Input: dimensioned drawing with shaded views. Units: mm. Origin: part minimum x, y, z. A direction names the side the tool comes from. Round coordinates to 2 decimals unless told otherwise and drop trailing zeros. Loops run counter-clockwise (first coordinate to the right, second up) from the corner with the lowest first, then second, coordinate; pieces in that order, holes last. Notation, with made-up numbers: M 69,60.25 L 94,60.25 A24 cw 94,95.25 Z; hole C 42,69.25 d6. An arc over 180 degrees is marked long. One line per item, written item: value.
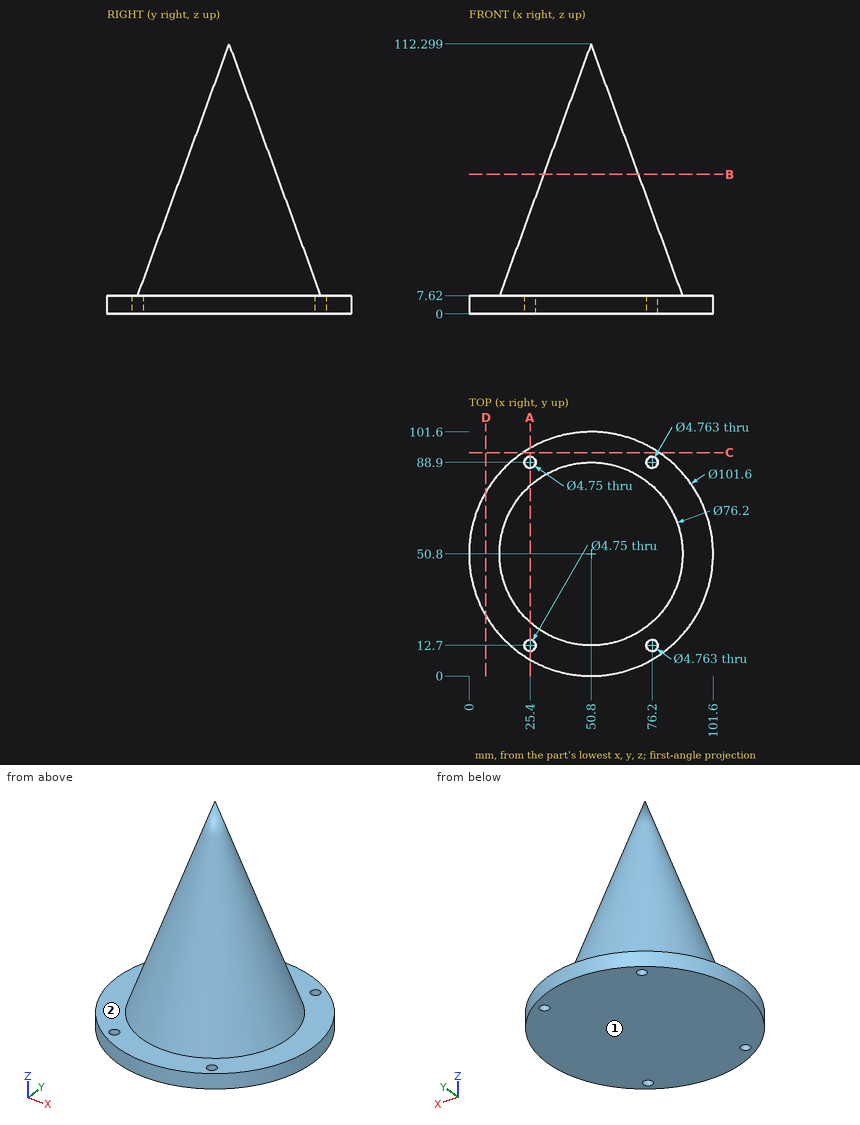
1. Reachability of the marked faces 1 and 2 from +Z, -Z, +X, -X, +Y, -Y: full face, straight path, thin tool, end or side. Return the list, or none.
Report:
face 1: -Z, +X, -X, +Y, -Y
face 2: +Z
2. Section query A-A (x = 25.4). Count the separate pieces of the cut face and the enclosed holes in it, and give its area (4 significant figures).
Report:
separate pieces: 3
enclosed holes: 0
area: 1,865 mm2
3. Section query D-D (x = 7). Return the cut outline in (y, z).
Report:
outline: M 25.07,0 L 76.53,0 L 76.53,7.62 L 25.07,7.62 Z
4. Pin query (flat end, axial travel): pin 1 (10 mm diameter, centred on y = 66.5, z = 30.5, fed in from +X); pin 2 (1.5 mm diameter, centred on x = 31.5, y = 11, fed in from -Z); pin 3 (12 mm diameter, centred on x = 70.5, z = 70, fed in from +Y); pin 4 (3 mm diameter, centred on x = 76.2, y = 12.7, fed in from +Z). Return the tip coordinate at first contact, or that it passes through.
Report:
pin 1: stops at x = 79.38
pin 2: stops at z = 0
pin 3: stops at y = 58.74
pin 4: passes through
5. Section query C-C (y = 93). Return the cut outline in (x, z).
Report:
outline: M 22.52,0 L 79.08,0 L 79.08,7.62 L 22.52,7.62 Z
6. Ray query, line 1 (X direction, y = 12, z = 2) (1 decimal); line 2 (X direction, y = 12.7, z = 4.5) (1 decimal); line 3 (Y direction, x = 25, z = 5). Return the intervals inside material, ascending. Write a range as [from, to].
Report:
line 1: x = [18, 23.1], [27.7, 73.9], [78.5, 83.6]
line 2: x = [17.2, 23], [27.8, 73.8], [78.6, 84.4]
line 3: y = [7.04, 10.36], [15.04, 86.56], [91.24, 94.56]
7. Section query B-B (z = 58). Return the cut outline in (x, y).
Report:
outline: C 50.8,50.8 d39.53
